Work out the finished part from the listing and answer in its coordinate system (mm). A direction names the side the tool comes from. Round coordinates to 2 decimals unless told otherwise and drop trailing zeros. Write each loop counter-clockwise with the first axis right and the second up, starting at its lowest first coordinate (ties: lowest second). Pieces come first, ordered by that corner, then holes. Notation, with made-up numbers: (6, 6) -> (21, 6) arc R25 cw to (21, 26) -> close; hole circle Ø9 at (12, 31). An arc over 180 degrees is marked (long way). Answer as a JSON object with one key per item and string values. Group by question number.
from build123d import *

# Parameters (mm, degrees)
BOSS_EXTRUDE1_DEPTH      = 13
BOSS_EXTRUDE1_DEPTH_BACK = 13
SKETCH1_R                = 90
SKETCH1_R_2              = 79
SKETCH5_R                = 3
CUT_EXTRUDE3_DEPTH       = 130.907659512
SKETCH6_W                = 20
SKETCH6_H                = 3
SKETCH6_W_2              = 3
SKETCH6_H_2              = 20
CUT_EXTRUDE4_DEPTH       = 130.907659512
SKETCH7_R                = 3
CUT_EXTRUDE5_DEPTH       = 199.244881708
SKETCH12_R               = 3
CUT_EXTRUDE8_DEPTH       = 199.244881715
SKETCH13_W               = 20
SKETCH13_H               = 3
SKETCH13_W_2             = 3
SKETCH13_H_2             = 20
CUT_EXTRUDE9_DEPTH       = 130.135587679


with BuildPart() as part:
    # Sketch1 → Boss-Extrude1 (new, two sides: drawn at the far end of the back side and taken through both)
    with BuildSketch(Plane(origin=(0, 0, 0), x_dir=(1, 0, 0), z_dir=(0, 1, 0)).offset(-BOSS_EXTRUDE1_DEPTH_BACK)):
        with Locations(Location((0, 0, 0), (0, 0, 270))):
            Circle(SKETCH1_R)
        with Locations(Location((0, 0, 0), (0, 0, 270))):
            Circle(SKETCH1_R_2, mode=Mode.SUBTRACT)
    extrude(amount=BOSS_EXTRUDE1_DEPTH + BOSS_EXTRUDE1_DEPTH_BACK)

    # Sketch5 → Cut-Extrude3 (cut, through all)
    with BuildSketch(Plane(origin=(0, 13, 0), x_dir=(1, 0, 0), z_dir=(0, 1, 0))):
        with Locations(Location((60.012131098, 60.012131098, 0), (0, 0, 270))):
            Circle(SKETCH5_R)
        with Locations(Location((60.012131098, -59.488914922, 0), (0, 0, 270))):
            Circle(SKETCH5_R)
        with Locations(Location((-59.488914922, -59.488914922, 0), (0, 0, 270))):
            Circle(SKETCH5_R)
        with Locations(Location((-59.488914922, 60.012131098, 0), (0, 0, 270))):
            Circle(SKETCH5_R)
    extrude(amount=-CUT_EXTRUDE3_DEPTH, mode=Mode.SUBTRACT)

    # Sketch6 → Cut-Extrude4 (cut, through all)
    with BuildSketch(Plane(origin=(0, 13, 0), x_dir=(1, 0, 0), z_dir=(0, 1, 0))):
        with Locations((0, -88.5)):
            Rectangle(SKETCH6_W, SKETCH6_H)
        with Locations((0, 88.5)):
            Rectangle(SKETCH6_W, SKETCH6_H)
        with Locations((88.5, 0)):
            Rectangle(SKETCH6_W_2, SKETCH6_H_2)
        with Locations((-88.5, 0)):
            Rectangle(SKETCH6_W_2, SKETCH6_H_2)
    extrude(amount=-CUT_EXTRUDE4_DEPTH, mode=Mode.SUBTRACT)

    # Sketch7 → Cut-Extrude5 (cut, through all)
    with BuildSketch(Plane.ZY.offset(87)):
        with Locations((0, 6)):
            Circle(SKETCH7_R)
        with Locations((0, -6)):
            Circle(SKETCH7_R)
    extrude(amount=-CUT_EXTRUDE5_DEPTH, mode=Mode.SUBTRACT)

    # Sketch12 → Cut-Extrude8 (cut, through all)
    with BuildSketch(Plane.XY.offset(87)):
        with Locations((0, 6)):
            Circle(SKETCH12_R)
        with Locations((0, -6)):
            Circle(SKETCH12_R)
    extrude(amount=-CUT_EXTRUDE8_DEPTH, mode=Mode.SUBTRACT)

    # Sketch13 → Cut-Extrude9 (cut, through all)
    with BuildSketch(Plane(origin=(0, 13, 0), x_dir=(1, 0, 0), z_dir=(0, 1, 0))):
        with Locations((0, -78.5)):
            Rectangle(SKETCH13_W, SKETCH13_H)
        with Locations((0, 78.5)):
            Rectangle(SKETCH13_W, SKETCH13_H)
        with Locations((-78.5, 0)):
            Rectangle(SKETCH13_W_2, SKETCH13_H_2)
        with Locations((78.5, 0)):
            Rectangle(SKETCH13_W_2, SKETCH13_H_2)
    extrude(amount=-CUT_EXTRUDE9_DEPTH, mode=Mode.SUBTRACT)


solid = part.part
1) A cutting plane is placed at D-D on z = -37. Determine the outline of the cut face in (x, y).
2) A cutting plane is placed at B-B on z = 0. Determine the outline of the cut face in (x, y).
3) Each of these flat-tipped pins is pushed along its axis until it touches: P1, Ø1.5, axis at x = 34, y = -9.5, coming from the -Z side; P2, Ø0.5, axis at x = 79.5, y = 4.5, coming from the +Z side; P3, Ø1.3, axis at y = 4, z = -79, coming from the -X side. Where does it stop, or does it pass through?
4) Straight lines are drawn through the part: L1, parallel to Y at x = 83, z = 0; L2, parallel to X at y = 4.25, z = -6.5. For each, find the intervals that lie inside material, in ascending order.
5) A tool of negligible diameter and unlimited length cuts with its end or side. For faces 5 (the face through (-83.55, 3.07, -0.65)), 6 (the face through (0, 0, 87)), 7 (the face through (0, 0, -80)), from which of +Z, -Z, +X, -X, +Y, -Y can it reach the whole face along a straight path? Write none if from no direction.
6) A cutting plane is placed at C-C on x = -18. Determine the outline of the cut face in (y, z).
7) A cutting plane is placed at A-A on x = 0. Determine the outline of the cut face in (y, z), plus the area to 3 significant figures.
8) For a pull along X with two mould halves and no side action, classify faces 1 (the face through (0, -3, 84)), 2 (the face through (87, 0, 0)), 3 (the face through (-72, 13, 33)), 4 (the face through (-87, 0, 0)) as released by +X, released by -X, zero draft, split by the parting line, or undercut.
Established:
{
 "1": {"outline": "(-82.04, -13) -> (-69.8, -13) -> (-69.8, 13) -> (-82.04, 13) -> close; (69.8, -13) -> (82.04, -13) -> (82.04, 13) -> (69.8, 13) -> close"},
 "2": {"outline": "(-87, -13) -> (-80, -13) -> (-80, -9) -> (-87, -9) -> close; (-87, -3) -> (-80, -3) -> (-80, 3) -> (-87, 3) -> close; (-87, 9) -> (-80, 9) -> (-80, 13) -> (-87, 13) -> close; (80, -13) -> (87, -13) -> (87, -9) -> (80, -9) -> close; (80, -3) -> (87, -3) -> (87, 3) -> (80, 3) -> close; (80, 9) -> (87, 9) -> (87, 13) -> (80, 13) -> close"},
 "3": {"P1": "stops at z = -83.63", "P2": "stops at z = 42.65", "P3": "stops at x = -44.29"},
 "4": {"L1": "y = -13 to -9, -3 to 3, 9 to 13", "L2": "x = -87 to -80, 80 to 87"},
 "5": {"face 5": "+X, -X", "face 6": "+Z, +Y, -Y", "face 7": "+Y, -Y"},
 "6": {"outline": "(-13, -88.18) -> (13, -88.18) -> (13, -76.92) -> (-13, -76.92) -> close; (-13, 76.92) -> (13, 76.92) -> (13, 88.18) -> (-13, 88.18) -> close"},
 "7": {"outline": "(-13, -87) -> (-9, -87) -> (-9, -80) -> (-13, -80) -> close; (-13, 80) -> (-9, 80) -> (-9, 87) -> (-13, 87) -> close; (-3, -87) -> (3, -87) -> (3, -80) -> (-3, -80) -> close; (-3, 80) -> (3, 80) -> (3, 87) -> (-3, 87) -> close; (9, -87) -> (13, -87) -> (13, -80) -> (9, -80) -> close; (9, 80) -> (13, 80) -> (13, 87) -> (9, 87) -> close", "area": "196 mm²"},
 "8": {"face 1": "undercut", "face 2": "released by +X", "face 3": "zero draft", "face 4": "released by -X"}
}
